from build123d import *

# Parameters (mm, degrees)
F1_DEPTH        = 50
F3_R            = 5.5
F4_DEPTH        = 10.5
F6_R            = 5.5
F7_DEPTH        = 10.5
F9_D            = 3.8
F9_CSINK_D      = 7.25
F9_CSINK_ANGLE  = 90
F11_D           = 3.8
F11_CSINK_D     = 7.25
F11_CSINK_ANGLE = 90


with BuildPart() as f1:
    # F0 (on Front) → F1 (new body)
    with BuildSketch(Plane.XZ):
        Polygon((3, 17.5), (0, 17.5), (0, 0), (17.5, 0), (17.5, 3), align=None)
    extrude(amount=-F1_DEPTH)

    # F3 (on offset) → F4 (cut)
    with BuildSketch(Plane.XY.offset(17.5)):
        with Locations((8.75, 40)):
            Circle(F3_R)
        with Locations((8.75, 10)):
            Circle(F3_R)
    extrude(amount=-F4_DEPTH, mode=Mode.SUBTRACT)

    # F6 (on offset) → F7 (cut)
    with BuildSketch(Plane.YZ.offset(17.5)):
        with Locations((25, 8.75)):
            Circle(F6_R)
    extrude(amount=-F7_DEPTH, mode=Mode.SUBTRACT)

    # F9 (through all)
    with Locations(Plane.XY.offset(7)):
        with Locations((8.75, 40), (8.75, 10)):
            CounterSinkHole(F9_D / 2, F9_CSINK_D / 2, counter_sink_angle=F9_CSINK_ANGLE)

    # F11 (through all)
    with Locations(Plane.YZ.offset(7)):
        with Locations((25, 8.75)):
            CounterSinkHole(F11_D / 2, F11_CSINK_D / 2, counter_sink_angle=F11_CSINK_ANGLE)


solid = f1.part
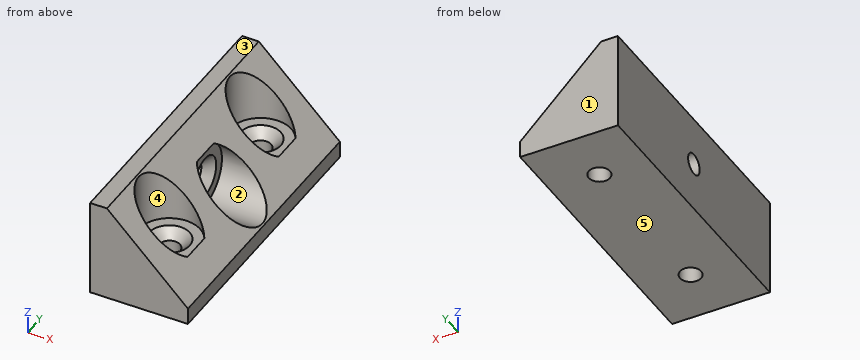
Here's how the part is built. I have some questions about the finished solid (model axes, mm). Face numbers are marked on the shaded views. A direction names the side the tool comes from. Round coordinates to 2 decimals unless told otherwise and drop trailing zeros. Write each loop counter-clockwise with the first axis right and the second up, starting at its lowest first coordinate (ties: lowest second). Pieces come first, ordered by that corner, then holes.
1. Suppose I cut it at C-C (z = 8.75). List the corners of the cut face in (x, y) for me (3 decimals).
2. Suppose I cut it at B-B (x = 3.75). List the corners of the cut face in (y, z) for me, and give its area (3 significant figures).
3. Will these pins go through, and if not, where does the flat tip stop? pin 1 Ø3 at (x, y) = (8, 20.5) entering from -Z; pin 2 Ø1 at (y, z) = (20.5, 7) entering from +X; pin 3 Ø3 at (y, z) = (23.5, 8) entering from +X; pin 4 Ø3 at (x, y) = (12.5, 43) entering from +Z.
4. If we mould it in two halves opening along Z, with no side actions, what happens to the marked faces 1, 2 and 3? For each: released by +Z, released by -Z, zero draft, split by the parting line, or undercut.
5. I need wall thicknesses on L1, parallel to Y at x = 8.75, z = 1.95; L2, parallel to Y at x = 9.5, z = 9.5; L3, parallel to Y at x = 7.5, z = 2.5. Which ranges of each line are inside material? Lowest first, please.
6. Suppose I cut it at D-D (x = 8.75). List the corners of the cut face in (y, z) for me (3 decimals), and give its area (3 significant figures).
7. Suppose I cut it at A-A (y = 40). List the corners of the cut face in (x, z) for me (3 decimals), and give its area (3 significant figures).
8. For the marked faces 4 and 5, which set-ups out of +Z, -Z, +X, -X, +Y, -Y let a thin tool reach every point of the face, with its end or its side?
Answer sheet:
1. outline: (0, 0) - (11.75, 0) - (11.75, 5.39) arc R5.5 cw (long way) to (11.75, 14.61) - (11.75, 19.5) - (7, 19.5) - (7, 21.375) - (5.275, 23.1) - (0, 23.1) - close; (0, 26.9) - (5.275, 26.9) - (7, 28.625) - (7, 30.5) - (11.75, 30.5) - (11.75, 35.39) arc R5.5 cw (long way) to (11.75, 44.61) - (11.75, 50) - (0, 50) - close
2. outline: (0, 0) - (50, 0) - (50, 16.75) - (42.29, 16.75) - (42.29, 7) - (37.71, 7) - (37.71, 16.75) - (12.29, 16.75) - (12.29, 7) - (7.71, 7) - (7.71, 16.75) - (0, 16.75) - close; hole circle Ø3.8 at (25, 8.75)
2. area: 737 mm2
3. pin 1: stops at z = 0
3. pin 2: stops at x = 7
3. pin 3: stops at x = 6.55
3. pin 4: stops at z = 8.48
4. face 1: zero draft
4. face 2: undercut
4. face 3: released by +Z
5. L1: y = 0 to 8.1, 11.9 to 38.1, 41.9 to 50
5. L2: y = 0 to 4.55, 15.45 to 19.55, 30.45 to 34.55, 45.45 to 50
5. L3: y = 0 to 8.57, 11.43 to 38.57, 41.43 to 50
6. outline: (0, 0) - (8.1, 0) - (8.1, 5.275) - (6.375, 7) - (4.5, 7) - (4.5, 11.75) - (0, 11.75) - close; (11.9, 0) - (38.1, 0) - (38.1, 5.275) - (36.375, 7) - (34.5, 7) - (34.5, 11.75) - (29.61, 11.75) arc R5.5 cw (long way) to (20.39, 11.75) - (15.5, 11.75) - (15.5, 7) - (13.625, 7) - (11.9, 5.275) - close; (41.9, 0) - (50, 0) - (50, 11.75) - (45.5, 11.75) - (45.5, 7) - (43.625, 7) - (41.9, 5.275) - close
6. area: 345 mm2
7. outline: (0, 0) - (6.85, 0) - (6.85, 5.275) - (5.125, 7) - (3.25, 7) - (3.25, 17.25) - (3, 17.5) - (0, 17.5) - close; (10.65, 0) - (17.5, 0) - (17.5, 3) - (13.5, 7) - (12.375, 7) - (10.65, 5.275) - close
7. area: 119 mm2
8. face 4: +Z
8. face 5: -Z, +X, -X, +Y, -Y
